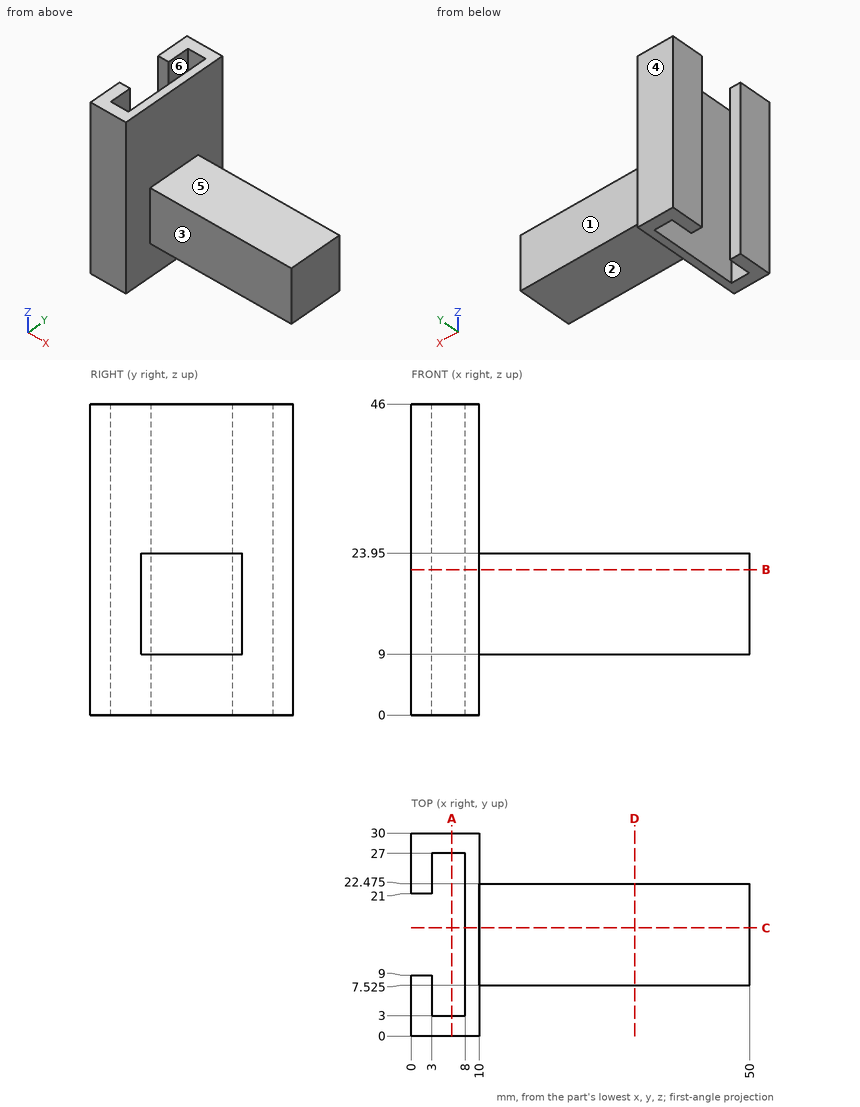
Geometry: see drawing. Coordinates: mm, zero at the bounding-box minimum. A direction names the side the tool comes from. Round coordinates to 2 decimals unless told otherwise and drop trailing zeros. Loops run counter-clockwise (first coordinate to the right, second up) from the corner with the lowest first, then second, coordinate; pieces in that order, holes last. Notation, with made-up numbers: (66, 62.25) - (84, 62.25) arc R25 cw to (84, 75.25) - close; hole circle Ø1 at (30.5, 42). An arc over 180 degrees is marked (long way). One line per item, written item: value. Start each with the question number.
(1) Section D-D, the plane x = 33. Return loops of the section in (y, z) (3 decimals).
(2) Contact query for flat-ended pins moving along their axis: P1, Ø4.5, axis at x = 27.5, y = 11.5, coming from the +Z side; P2, Ø2.5, axis at x = 1, z = 12, coming from the -Y side; P3, Ø16.5, axis at x = 35.5, y = 13.5, coming from the -Z side; P4, Ø10, axis at x = 21, z = 21, coming from the +Y side (3 decimals). Output: stop coordinate, or through.
(3) Section C-C, the plane y = 16. Return loops of the section in (x, z), plus the area to 3 significant figures.
(4) Section B-B, the plane z = 21.5. Return loops of the section in (x, y) (3 decimals).
(5) Section A-A, the plane x = 6. Return loops of the section in (y, z), plus the area to 3 significant figures.
(6) Ray query, line 1 (X direction, y = 4.75, z = 29); line 2 (X direction, y = 21.5, z = 16.5); line 3 (Y direction, x = 7.5, z = 15). Return the intervals inside material, ascending. Write a range as [from, to].
(7) Draft query along Y for the marked faces 4, 5 and 6. Return one class per face: +Y half, -Y half, draft (parallel to the pull), parting line (faces both ways), or undercut.
(8) Access query for the marked faces 1, 2 and 3. Directions: +Z, -Z, +X, -X, +Y, -Y. A direction counts if a zero-diameter tool reaches every point of the face in a straight line with its end or side. Return the directions, or none.
Results below:
1. outline: (7.525, 9) - (22.475, 9) - (22.475, 23.95) - (7.525, 23.95) - close
2. P1: z = 23.95
2. P2: y = 0
2. P3: z = 9
2. P4: y = 22.475
3. outline: (8, 0) - (10, 0) - (10, 9) - (50, 9) - (50, 23.95) - (10, 23.95) - (10, 46) - (8, 46) - close
3. area: 690 mm^2
4. outline: (0, 0) - (10, 0) - (10, 7.525) - (50, 7.525) - (50, 22.475) - (10, 22.475) - (10, 30) - (0, 30) - (0, 21) - (3, 21) - (3, 27) - (8, 27) - (8, 3) - (3, 3) - (3, 9) - (0, 9) - close
5. outline: (0, 0) - (3, 0) - (3, 46) - (0, 46) - close; (27, 0) - (30, 0) - (30, 46) - (27, 46) - close
5. area: 276 mm^2
6. line 1: [0, 3], [8, 10]
6. line 2: [0, 3], [8, 50]
6. line 3: [0, 3], [27, 30]
7. face 4: +Y half
7. face 5: draft
7. face 6: undercut
8. face 1: +Z, -Z, +X, +Y
8. face 2: -Z, +X, +Y, -Y
8. face 3: +Z, -Z, +X, -Y
